Input: part model. Units: mm. Frame: model coordinates. A direction names the side the tool comes from. Round coordinates to 2 decimals unless told otherwise and drop trailing zeros. Order: outer loops, then holes, each group sorted by start corner. A loop starts at its lowest first (then second) coordinate and runs counter-clockwise, first axis right, second up. Notation, with made-up numbers: (81, 42) -> (93, 42) arc R17 ccw to (93, 75) -> close; hole circle Ø9 at (82.5, -10). An arc over 180 degrees is marked (long way). Use a Markdown table: item, result.
from build123d import *

# Parameters (mm, degrees)
F0_R     = 457.2
F0_R_2   = 254
F1_DEPTH = 508
F2_R     = 457.2
F2_R_2   = 419.1
F3_DEPTH = 203.2
F4_R     = 457.2
F4_R_2   = 355.6
F5_DEPTH = 203.2


with BuildPart() as f1:
    # F0 (on Top) → F1 (new body)
    with BuildSketch(Plane.XY):
        Circle(F0_R)
        Circle(F0_R_2, mode=Mode.SUBTRACT)
    extrude(amount=F1_DEPTH)

    # F2 (on face) → F3 (cut)
    with BuildSketch(Plane.XY.offset(508)):
        Circle(F2_R)
        Circle(F2_R_2, mode=Mode.SUBTRACT)
    extrude(amount=-F3_DEPTH, mode=Mode.SUBTRACT)

    # F4 (on face) → F5 (cut)
    with BuildSketch(Plane.XY):
        Circle(F4_R)
        Circle(F4_R_2, mode=Mode.SUBTRACT)
    extrude(amount=F5_DEPTH, mode=Mode.SUBTRACT)


solid = f1.part
1) Cut plane C-C on z = 239. Return loops of the section in (x, y).
Results found:
| item | result |
|---|---|
| outline | circle Ø914.4 at (0, 0); hole circle Ø508 at (0, 0) |
2) Pin query (flat end, axial travel): pin 1 Ø10 at (y, z) = (-186, 371) entering from -X; pin 2 Ø12 at (y, z) = (329.5, 410) entering from +X; pin 3 Ø5 at (y, z) = (211, 400.5) entering from +X. Return the tip coordinate at first contact, or that it passes through.
Results found:
| item | result |
|---|---|
| pin 1 | stops at x = -378 |
| pin 2 | stops at x = 266.44 |
| pin 3 | stops at x = 363.56 |
3) Cut plane D-D on x = -316. Return loops of the section in (y, z), and give its area (3 significant figures).
Results found:
| item | result |
|---|---|
| outline | (-330.42, 203.2) -> (-163.08, 203.2) -> (-163.08, 0) -> (163.08, 0) -> (163.08, 203.2) -> (330.42, 203.2) -> (330.42, 304.8) -> (275.3, 304.8) -> (275.3, 508) -> (-275.3, 508) -> (-275.3, 304.8) -> (-330.42, 304.8) -> close |
| area | 245,000 mm² |
4) Line query: L1, parallel to Y at x = 0, z = 135; L2, parallel to X at y = 7, z = 152; L3, parallel to Z at x = -155, y = -373. Output: solid intervals per line, ascending. Write a range as [from, to].
Results found:
| item | result |
|---|---|
| L1 | y = [-355.6, -254], [254, 355.6] |
| L2 | x = [-355.53, -253.9], [253.9, 355.53] |
| L3 | z = [203.2, 508] |
5) Pull-direction query (Y, two-part tool) for faces 4 (the cylindrical face through (-456.758, 20.102, 253.289)), 5 (the flat face through (-242, 84, 0)), 6 (the cylindrical face through (-55.06, -247.96, 250.44)); classes: +Y half, -Y half, draft (parallel to the pull), parting line (faces both ways), or undercut.
Results found:
| item | result |
|---|---|
| face 4 | parting line |
| face 5 | draft |
| face 6 | undercut |
6) Cut plane A-A on x = 0. Return loops of the section in (y, z), and give its area (3 significant figures).
Results found:
| item | result |
|---|---|
| outline | (-457.2, 203.2) -> (-355.6, 203.2) -> (-355.6, 0) -> (-254, 0) -> (-254, 508) -> (-419.1, 508) -> (-419.1, 304.8) -> (-457.2, 304.8) -> close; (254, 0) -> (355.6, 0) -> (355.6, 203.2) -> (457.2, 203.2) -> (457.2, 304.8) -> (419.1, 304.8) -> (419.1, 508) -> (254, 508) -> close |
| area | 150,000 mm² |
7) Set-up query: faces 1 (the cylindrical face through (339.18, 106.81, 100.18)), 2 (the flat face through (201, -370, 304.8)), 3 (the flat face through (180, -180, 508)). Return all of +Z, -Z, +X, -X, +Y, -Y with unobstructed straight access to the full face (end or side cutting, diameter ignored); none if empty.
Results found:
| item | result |
|---|---|
| face 1 | -Z |
| face 2 | +Z |
| face 3 | +Z, +X, -X, +Y, -Y |
